from build123d import *

# Parameters (mm, degrees)
F1_W     = 27
F1_H     = 43.8
F1_R     = 1.5
F1_H_2   = 10
F2_DEPTH = 28
F3_R     = 1.75
F4_DEPTH = 63.801
F5_W     = 47.8
F5_H     = 24
F6_DEPTH = 27.001


with BuildPart() as f2:
    # F1 (on Top) → F2 (new body)
    with BuildSketch(Plane.XY):
        Rectangle(F1_W, F1_H)
        with Locations((-10, -10)):
            Circle(F1_R, mode=Mode.SUBTRACT)
        with Locations((10, -10)):
            Circle(F1_R, mode=Mode.SUBTRACT)
        with Locations((-10, 10)):
            Circle(F1_R, mode=Mode.SUBTRACT)
        with Locations((10, 10)):
            Circle(F1_R, mode=Mode.SUBTRACT)
        with Locations((0, 26.9)):
            Rectangle(F1_W, F1_H_2)
        with Locations((0, -26.9)):
            Rectangle(F1_W, F1_H_2)
    extrude(amount=F2_DEPTH)

    # F3 (on face) → F4 (cut, through all)
    with BuildSketch(Plane(origin=(0, 31.9, 0), x_dir=(-1, 0, 0), z_dir=(0, 1, 0))):
        with Locations((0, 23.697)):
            Circle(F3_R)
        with Locations((0, 4.302)):
            Circle(F3_R)
    extrude(amount=-F4_DEPTH, mode=Mode.SUBTRACT)

    # F5 (on face) → F6 (cut, through all)
    with BuildSketch(Plane(origin=(-13.5, 0, 0), x_dir=(0, -1, 0), z_dir=(-1, 0, 0))):
        with Locations((0, 16)):
            Rectangle(F5_W, F5_H)
    extrude(amount=-F6_DEPTH, mode=Mode.SUBTRACT)


solid = f2.part
Source: CAD feature listing. Evaluate the final solid. Frame: model axes, mm. A direction names the side the tool comes from. Round coordinates to 2 decimals unless told otherwise and drop trailing zeros. Write each loop counter-clockwise with the first axis right and the second up, starting at its lowest first coordinate (ties: lowest second). Pieces come first, ordered by that corner, then holes. Notation, with made-up numbers: M 32,-21.5 L 57,-21.5 A32 cw 57,7.5 Z; hole C -17,9 d1. An arc over 180 degrees is marked long. One line per item, written item: value. Start each with the question number.
Item 1: Section query C-C (z = 18.75). Return the cut outline in (x, y).
Item 2: Set-up query: faces 1 (the flat face through (0, 23.9, 16)), 2 (the cylindrical face through (0.4, 0.4, 2.6)). Return all of +Z, -Z, +X, -X, +Y, -Y with unobstructed straight access to the full face (end or side cutting, diameter ignored); none if empty.
Item 3: Ray query, L1, parallel to X at y = -10, z = 2.1; L2, parallel to Y at x = 10, z = 0.85; L3, parallel to Z at x = 0, y = 28.25. Return the intervals inside material, ascending. Write a range as from..to.
Item 4: Pin query (flat end, axial travel): pin 1 (3.5 mm diameter, centred on x = 9, y = -4.5, fed in from +Z). Return the tip coordinate at first contact, or that it passes through.
Item 5: Section query A-A (x = 0). Return the cut outline in (y, z), plus the area to 3 significant figures.
Item 6: Section query D-D (y = 10). Return the cut outline in (x, z).
Item 7: Section query B-B (x = 10). Return the cut outline in (y, z), plus the area to 3 significant figures.
Item 8: Mould query, pull axis Y, two halves, no side actions, for faces 3 (the cylindrical face through (8.8, 9.1, 2)), 4 (the flat face through (-13.5, 0.1, 3.6)), 5 (the flat face through (0, 31.9, 14)), 6 (the flat face through (0, -31.9, 14)). Classes: pulls with the +Y half, pulls with the -Y half, needs draft (parallel to the pull), parting line crosses it, or undercut.
Result set:
1. outline: M -13.5,-31.9 L 13.5,-31.9 L 13.5,-23.9 L -13.5,-23.9 Z; M -13.5,23.9 L 13.5,23.9 L 13.5,31.9 L -13.5,31.9 Z
2. face 1: +Z, +X, -X
2. face 2: +Y, -Y
3. L1: x = -13.5..-11.5, -8.5..8.5, 11.5..13.5
3. L2: y = -31.9..-11.5, -8.5..8.5, 11.5..31.9
3. L3: z = 0..2.55, 6.05..21.95, 25.45..28
4. pin 1: stops at z = 4
5. outline: M -31.9,0 L 31.9,0 L 31.9,2.55 L -31.9,2.55 Z; M -31.9,6.05 L -23.9,6.05 L -23.9,21.95 L -31.9,21.95 Z; M -31.9,25.45 L -23.9,25.45 L -23.9,28 L -31.9,28 Z; M 23.9,6.05 L 31.9,6.05 L 31.9,21.95 L 23.9,21.95 Z; M 23.9,25.45 L 31.9,25.45 L 31.9,28 L 23.9,28 Z
5. area: 458 mm²
6. outline: M -13.5,0 L -11.5,0 L -11.5,4 L -13.5,4 Z; M -8.5,0 L 8.5,0 L 8.5,4 L 1.72,4 A1.75 cw -1.72,4 L -8.5,4 Z; M 11.5,0 L 13.5,0 L 13.5,4 L 11.5,4 Z
7. outline: M -31.9,0 L -11.5,0 L -11.5,4 L -23.9,4 L -23.9,28 L -31.9,28 Z; M -8.5,0 L 8.5,0 L 8.5,4 L -8.5,4 Z; M 11.5,0 L 31.9,0 L 31.9,28 L 23.9,28 L 23.9,4 L 11.5,4 Z
7. area: 615 mm²
8. face 3: undercut
8. face 4: needs draft
8. face 5: pulls with the +Y half
8. face 6: pulls with the -Y half
